Check sheet for the modelled part. Datum: model origin and axes. Units: mm. A direction names the side the tool comes from. Round coordinates to 2 decimals unless told otherwise and drop trailing zeros. Order: outer loops, then holes, each group sorted by start corner. A loop starts at its lowest first (then second) coordinate and runs counter-clockwise, first axis right, second up. Notation, with made-up numbers: M 17.5,-5 L 25.5,-5 A26 ccw 25.5,27 Z; hole C 18.25,63 d10. An arc over 180 degrees is marked long. One line per item, written item: value. Start each with the question number.
(1) Cross-section at D-D, the plane x = 33.15. Enter the section's corners in (y, z) (3 decimals).
(2) Release check for a two-part mould opening along Z. For faces 3 (the face through (31, 20, 0)), 4 (the face through (50.8, 48, 15)), 5 (the face through (28.43, 49.19, 42.23)) record: released by +Z, released by -Z, zero draft, split by the parting line, or undercut.
(3) Cross-section at A-A, the plane x = 40.9. Enter the section's corners in (y, z) (3 decimals).
(4) Depth check by flat-ended pin: pin 1 Ø2 at (x, y) = (42.5, 40) entering from +Z (3 decimals); pin 2 Ø12 at (x, z) = (14.5, 48.5) entering from -Y (3 decimals). Enter the tip coordinate at first touch or a pass-through.
(5) Thickness scan on L1, parallel to Z at x = 25.4, y = 48.35 (3 decimals); L2, parallel to X at y = 19, z = 2; L3, parallel to X at y = 26, z = 2. Record the ranges inside material, lowest first.
(6) Access from +Z, -Z, +X, -X, +Y, -Y to the whole of each face (thin tool, end or side, straight path). Record for faces 1 (the face through (34.536, 5.052, 1.565)), 2 (the face through (25, 47.625, 28)).
(7) Cross-section at B-B, the plane x = 25.4. Enter the section's corners in (y, z) (3 decimals), and give its area (3 significant figures).
(8) Cross-section at C-C, the plane y = 24.5. Enter the section's corners in (x, z) (3 decimals).
from build123d import *

# Parameters (mm, degrees)
SKETCH1_W           = 50.8
SKETCH1_H           = 50.8
SKETCH1_R           = 6.5
SKETCH1_R_2         = 1.5
BOSS_EXTRUDE1_DEPTH = 3.175
SKETCH2_W           = 50.8
SKETCH2_H           = 3.175
BOSS_EXTRUDE2_DEPTH = 50.8
SKETCH3_R           = 3.175
CUT_EXTRUDE1_DEPTH  = 4.175


with BuildPart() as part:
    # Sketch1 → Boss-Extrude1 (new body)
    with BuildSketch(Plane.XY):
        with Locations((25.4, 25.4)):
            Rectangle(SKETCH1_W, SKETCH1_H)
        with Locations((25.4, 26.05)):
            Circle(SKETCH1_R, mode=Mode.SUBTRACT)
        with Locations((9.9, 19.05)):
            Circle(SKETCH1_R_2, mode=Mode.SUBTRACT)
        with Locations((40.9, 19.05)):
            Circle(SKETCH1_R_2, mode=Mode.SUBTRACT)
        with Locations((33.15, 5.626606241)):
            Circle(SKETCH1_R_2, mode=Mode.SUBTRACT)
        with Locations((17.65, 5.626606241)):
            Circle(SKETCH1_R_2, mode=Mode.SUBTRACT)
        with Locations((17.65, 32.473393759)):
            Circle(SKETCH1_R_2, mode=Mode.SUBTRACT)
        with Locations((33.15, 32.473393759)):
            Circle(SKETCH1_R_2, mode=Mode.SUBTRACT)
    extrude(amount=BOSS_EXTRUDE1_DEPTH)

    # Sketch2 → Boss-Extrude2 (add)
    with BuildSketch(Plane.XY.offset(3.175)):
        with Locations((25.4, 49.2125)):
            Rectangle(SKETCH2_W, SKETCH2_H)
    extrude(amount=BOSS_EXTRUDE2_DEPTH)

    # Sketch3 → Cut-Extrude1 (cut, through all)
    with BuildSketch(Plane.XZ.offset(-47.625)):
        with Locations((25.4, 41.275)):
            Circle(SKETCH3_R)
        with Locations((25.4, 22.225)):
            Circle(SKETCH3_R)
    extrude(amount=-CUT_EXTRUDE1_DEPTH, mode=Mode.SUBTRACT)


solid = part.part
Values found:
1. outline: M 0,0 L 4.127,0 L 4.127,3.175 L 0,3.175 Z; M 7.127,0 L 30.973,0 L 30.973,3.175 L 7.127,3.175 Z; M 33.973,0 L 50.8,0 L 50.8,53.975 L 47.625,53.975 L 47.625,3.175 L 33.973,3.175 Z
2. face 3: released by -Z
2. face 4: zero draft
2. face 5: undercut
3. outline: M 0,0 L 17.55,0 L 17.55,3.175 L 0,3.175 Z; M 20.55,0 L 50.8,0 L 50.8,53.975 L 47.625,53.975 L 47.625,3.175 L 20.55,3.175 Z
4. pin 1: z = 3.175
4. pin 2: y = 47.625
5. L1: 0 to 19.05, 25.4 to 38.1, 44.45 to 53.975
5. L2: 0 to 8.4, 11.4 to 39.4, 42.4 to 50.8
5. L3: 0 to 18.9, 31.9 to 50.8
6. face 1: +Z, -Z
6. face 2: +Z, +X, -X, -Y
7. outline: M 0,0 L 19.55,0 L 19.55,3.175 L 0,3.175 Z; M 32.55,0 L 50.8,0 L 50.8,19.05 L 47.625,19.05 L 47.625,3.175 L 32.55,3.175 Z; M 47.625,25.4 L 50.8,25.4 L 50.8,38.1 L 47.625,38.1 Z; M 47.625,44.45 L 50.8,44.45 L 50.8,53.975 L 47.625,53.975 Z
7. area: 241 mm^2
8. outline: M 0,0 L 19.088,0 L 19.088,3.175 L 0,3.175 Z; M 31.712,0 L 50.8,0 L 50.8,3.175 L 31.712,3.175 Z
